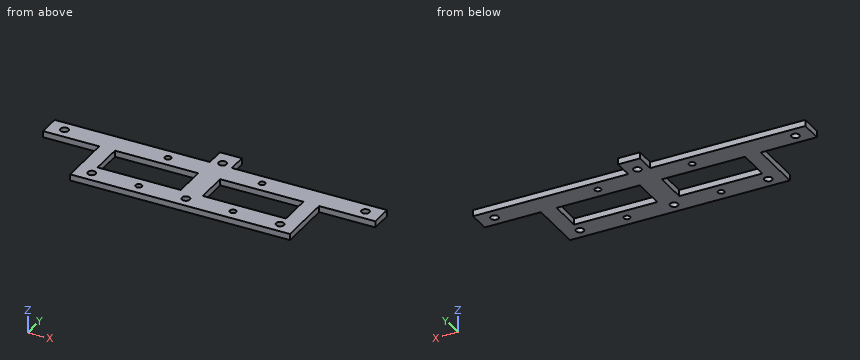
```python
from build123d import *

# Parameters (mm, degrees)
SKETCH1_R           = 2.5
SKETCH1_R_2         = 2
SKETCH1_W           = 10
SKETCH1_H           = 20.877946607
SKETCH1_W_2         = 140
SKETCH1_H_2         = 14
BOSS_EXTRUDE1_DEPTH = 4


with BuildPart() as part:
    # Sketch1 → Boss-Extrude1 (new body)
    # profile 1 of 6: a face of its own
    with BuildSketch(Plane.XY):
        Polygon((-105.826370741, 27.877946607), (-70, 27.877946607), (-60, 27.877946607), (-7, 27.877946607), (-7, 41.877946607), (-105.826370741, 41.877946607), align=None)
        with Locations((-95.826370741, 34.877946607)):
            Circle(SKETCH1_R, mode=Mode.SUBTRACT)
        with Locations((-30, 34.877946607)):
            Circle(SKETCH1_R_2, mode=Mode.SUBTRACT)
    # profile 2 of 6: a face of its own
    with BuildSketch(Plane.XY):
        with Locations((-65, 17.438973303)):
            Rectangle(SKETCH1_W, SKETCH1_H)
    # profile 3 of 6: a face of its own
    with BuildSketch(Plane.XY):
        Rectangle(SKETCH1_W_2, SKETCH1_H_2)
        with Locations((30, 0)):
            Circle(SKETCH1_R_2, mode=Mode.SUBTRACT)
        with Locations((-30, 0)):
            Circle(SKETCH1_R_2, mode=Mode.SUBTRACT)
        with Locations((-60, 0)):
            Circle(SKETCH1_R, mode=Mode.SUBTRACT)
        Circle(SKETCH1_R, mode=Mode.SUBTRACT)
        with Locations((60, 0)):
            Circle(SKETCH1_R, mode=Mode.SUBTRACT)
    # profile 4 of 6: a face of its own
    with BuildSketch(Plane.XY):
        Polygon((-7, 27.877946607), (-7, 7), (7, 7), (7, 27.877946607), (7, 41.877946607), (7, 54), (-7, 54), (-7, 41.877946607), align=None)
        with Locations((0, 44)):
            Circle(SKETCH1_R, mode=Mode.SUBTRACT)
    # profile 5 of 6: a face of its own
    with BuildSketch(Plane.XY):
        Polygon((7, 41.877946607), (7, 27.877946607), (60, 27.877946607), (70, 27.877946607), (105.826370741, 27.877946607), (105.826370741, 41.877946607), align=None)
        with Locations((30, 34.877946607)):
            Circle(SKETCH1_R_2, mode=Mode.SUBTRACT)
        with Locations((95.826370741, 34.877946607)):
            Circle(SKETCH1_R, mode=Mode.SUBTRACT)
    # profile 6 of 6: a face of its own
    with BuildSketch(Plane.XY):
        with Locations((65, 17.438973303)):
            Rectangle(SKETCH1_W, SKETCH1_H)
    extrude(amount=BOSS_EXTRUDE1_DEPTH)


solid = part.part
```
The model under review builds one solid part; all positions refer to its coordinate system, in mm. Give positions to 0.01 mm unless a question says otherwise; leave off trailing zeros. Write each loop counter-clockwise with the first axis right and the second up, starting at its lowest first coordinate (ties: lowest second). Pieces come first, ordered by that corner, then holes.
(1) For P1, Ø8, axis at x = 0, y = 44, coming from the +Z side; P2, Ø1.5, axis at x = 19, z = 3.5, coming from the +Y side; P3, Ø2, axis at y = 8.5, z = 1.5, coming from the -X side; P4, Ø1.2, axis at x = 84, z = 2.5, coming from the -Y side, all flat-tipped, find the tip position at first contact; note any pin that passes through.
(2) Consider section C-C, the plane y = 14.5. Give the boundary of the cut face in (x, z), and give its area (3 significant figures).
(3) To check wall thickness, follow L1, parallel to X at y = 26.5, z = 3.75; L2, parallel to Y at x = -34, z = 0.65; L3, parallel to Y at x = 61.5, z = 3.45. State the ranges of each line that lie inside material, in increasing order.
(4) Consider section D-D, the plane z = 2.95. Give the number of separate pieces and of enclosed holes in the cut face, and give its area (3 significant figures).
(5) Consider section B-B, the plane y = 0. Give the boundary of the cut face in (x, z), and give its area (3 significant figures).
(6) Consider section A-A, the plane x = 38.5. Give the boundary of the cut face in (y, z).
Returned:
1. P1: stops at z = 4
1. P2: stops at y = 41.88
1. P3: stops at x = -70
1. P4: stops at y = 27.88
2. outline: (-70, 0) - (-60, 0) - (-60, 4) - (-70, 4) - close; (-7, 0) - (7, 0) - (7, 4) - (-7, 4) - close; (60, 0) - (70, 0) - (70, 4) - (60, 4) - close
2. area: 136 mm2
3. L1: x = -70 to -60, -7 to 7, 60 to 70
3. L2: y = -7 to 7, 27.88 to 41.88
3. L3: y = -7 to -2, 2 to 41.88
4. separate pieces: 1
4. enclosed holes: 12
4. area: 5,630 mm2
5. outline: (-70, 0) - (-62.5, 0) - (-62.5, 4) - (-70, 4) - close; (-57.5, 0) - (-32, 0) - (-32, 4) - (-57.5, 4) - close; (-28, 0) - (-2.5, 0) - (-2.5, 4) - (-28, 4) - close; (2.5, 0) - (28, 0) - (28, 4) - (2.5, 4) - close; (32, 0) - (57.5, 0) - (57.5, 4) - (32, 4) - close; (62.5, 0) - (70, 0) - (70, 4) - (62.5, 4) - close
5. area: 468 mm2
6. outline: (-7, 0) - (7, 0) - (7, 4) - (-7, 4) - close; (27.88, 0) - (41.88, 0) - (41.88, 4) - (27.88, 4) - close
